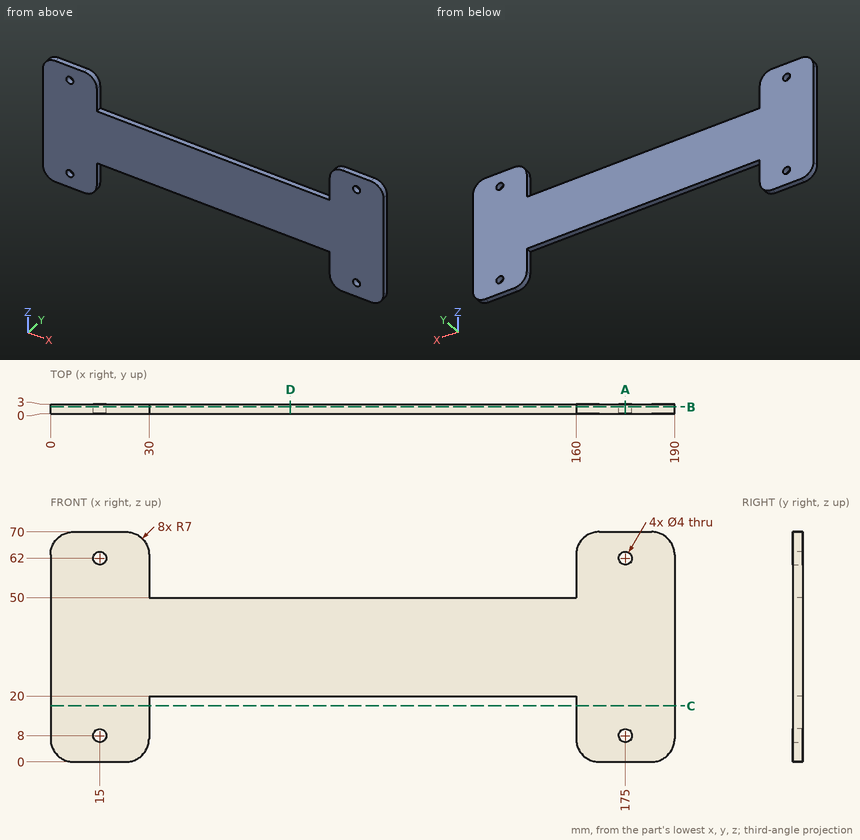
Study the drawing (mm; zero at the part's minimum x, y, z) and answer. Coordinates: 2 decimals unless noted, no trailing zeros. Write each loop counter-clockwise with the first axis right and the second up, starting at its lowest first coordinate (ties: lowest second). Pieces come first, ordered by that corner, then holes. Notation, with made-up numbers: M -28.75,2.25 L 24.25,2.25 A13 ccw 24.25,13.25 Z; hole C -34.5,76 d10. An arc over 180 degrees is marked long. Use a Markdown table: item, result. Add a question column.
1. Section A-A (x = 175) is taken. Give the vertices of the cut face in (y, z), plus the area to 3 significant figures.
2. Section C-C (z = 17) is taken. Give the vertices of the cut face in (x, y), plus the area to 3 significant figures.
3. Given P1, Ø0.9, axis at x = 123, y = 1, coming from the +Z side; P2, Ø1, axis at x = 163, y = 1, coming from the -Z side; P3, Ø3, axis at x = 175, z = 8, coming from the +Y side, each flat-ended and moving along its own axis, determine where each tip first touches the part or whether it passes through.
4. Section D-D (x = 73) is taken. Give the vertices of the cut face in (y, z).
5. Straight lines are drawn through the part: line 1 along Z through (x, y) = (175, 1.8); line 2 along X through (y, z) = (1.05, 8); line 3 along Z through (x, y) = (84, 1.1). For each, find the intervals that lie inside material, in ascending order. Write a range as [from, to].
6. Section B-B (y = 2.15) is taken. Give the vertices of the cut face in (x, z), plus the area to 3 significant figures.
Data:
| question | item | result |
|---|---|---|
| 1 | outline | M 0,0 L 3,0 L 3,6 L 0,6 Z; M 0,10 L 3,10 L 3,60 L 0,60 Z; M 0,64 L 3,64 L 3,70 L 0,70 Z |
| 1 | area | 186 mm2 |
| 2 | outline | M 0,0 L 30,0 L 30,3 L 0,3 Z; M 160,0 L 190,0 L 190,3 L 160,3 Z |
| 2 | area | 180 mm2 |
| 3 | P1 | stops at z = 50 |
| 3 | P2 | stops at z = 0.94 |
| 3 | P3 | passes through |
| 4 | outline | M 0,20 L 3,20 L 3,50 L 0,50 Z |
| 5 | line 1 | z = [0, 6], [10, 60], [64, 70] |
| 5 | line 2 | x = [0, 13], [17, 30], [160, 173], [177, 190] |
| 5 | line 3 | z = [20, 50] |
| 6 | outline | M 0,7 A7 ccw 7,0 L 23,0 A7 ccw 30,7 L 30,20 L 160,20 L 160,7 A7 ccw 167,0 L 183,0 A7 ccw 190,7 L 190,63 A7 ccw 183,70 L 167,70 A7 ccw 160,63 L 160,50 L 30,50 L 30,63 A7 ccw 23,70 L 7,70 A7 ccw 0,63 Z; hole C 15,8 d4; hole C 15,62 d4; hole C 175,8 d4; hole C 175,62 d4 |
| 6 | area | 7,970 mm2 |
